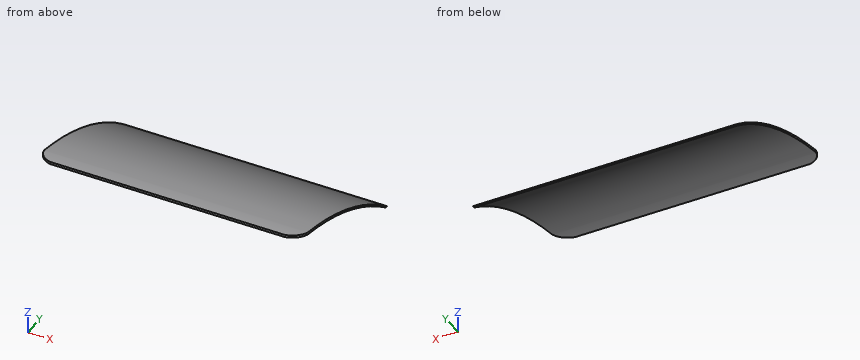
from build123d import *

# Parameters (mm, degrees)
F1_DEPTH      = 154.94
F1_DEPTH_BACK = 154.94
F3_DEPTH      = 186.182


with BuildPart() as f1:
    # F0 (on Right) → F1 (new body, two sides)
    with BuildSketch(Plane.YZ) as f1_sk:
        with BuildLine():
            ThreePointArc((-188.7878807099, 75.1623316368), (-89.2907214559, 50.3991008102), (0, 0))
            Line((0, 0), (2.794, 0))
            ThreePointArc((2.794, 0), (-87.6056719262, 52.227498147), (-188.7878807099, 77.9563316368))
            Line((-188.7878807099, 77.9563316368), (-188.7878807099, 75.1623316368))
        make_face()
    extrude(amount=-F1_DEPTH)
    extrude(f1_sk.sketch, amount=F1_DEPTH_BACK)

    # F2 (on Top) → F3 (cut)
    with BuildSketch(Plane.XY):
        with BuildLine():
            ThreePointArc((-126.7025372224, -188.7878807099), (-147.6240234131, -183.5115430003), (-154.94, -163.2131487131))
            Line((-154.94, -163.2131487131), (-161.3427400589, -163.2131487131))
            Line((-161.3427400589, -163.2131487131), (-161.3427400589, -196.9332418511))
            Line((-161.3427400589, -196.9332418511), (-120.7653358579, -196.9332418511))
            Line((-120.7653358579, -196.9332418511), (-126.7025372224, -188.7878807099))
        make_face()
        with BuildLine():
            Line((126.7025372224, -188.7878807099), (120.7653358579, -196.9332418511))
            Line((120.7653358579, -196.9332418511), (161.3427400589, -196.9332418511))
            Line((161.3427400589, -196.9332418511), (161.3427400589, -163.2131487131))
            Line((161.3427400589, -163.2131487131), (154.94, -163.2131487131))
            ThreePointArc((154.94, -163.2131487131), (147.6240234131, -183.5115430003), (126.7025372224, -188.7878807099))
        make_face()
    extrude(amount=F3_DEPTH, mode=Mode.SUBTRACT)


solid = f1.part
Model file for the job. Use its own axes, mm. Give positions to 0.01 mm unless a question says otherwise; leave off trailing zeros. Loops run counter-clockwise (first coordinate to the right, second up) from the corner with the lowest first, then second, coordinate; pieces in that order, holes last. Notation, with made-up numbers: (72.5, 17.25) -> (117.5, 17.25) arc R22 cw to (117.5, 24.25) -> close; hole circle Ø3 at (74, 51.5). An arc over 180 degrees is marked (long way). Use a Markdown table: item, result. Add a question column.
(1) Slice it at A-A on y = -71. List the corners of the cut face in (x, z).
(2) Slice it at B-B on x = -36. List the corners of the cut face in (y, z).
(3) Drop flat-ended pins along their axis: pin 1 Ø4 at (x, y) = (-29, -137) entering from -Z; pin 2 Ø10 at (x, y) = (-102, -158.5) entering from -Z; pin 3 Ø3 at (x, z) = (-59.5, 16.5) entering from -Y; pin 4 Ø4 at (y, z) = (-99, 59) entering from -X. Give the stop position or say it passes through.
(4) Wall check: line 1 along Z through (x, y) = (41, -177); line 2 along Y through (x, z) = (73, 39.5); line 3 along Z through (x, y) = (-85.5, -102). Give the ranges that are in metal, low to high.
Filled sheet:
| question | item | result |
|---|---|---|
| 1 | outline | (-154.94, 42.56) -> (154.94, 42.56) -> (154.94, 45.01) -> (-154.94, 45.01) -> close |
| 2 | outline | (-188.79, 75.16) arc R381 cw to (0, 0) -> (2.79, 0) arc R381 ccw to (-188.79, 77.96) -> close |
| 3 | pin 1 | z = 65.33 |
| 3 | pin 2 | z = 69.62 |
| 3 | pin 3 | y = -25.9 |
| 3 | pin 4 | through |
| 4 | line 1 | 73.69 to 76.45 |
| 4 | line 2 | -64.51 to -59.62 |
| 4 | line 3 | 55.2 to 57.75 |
